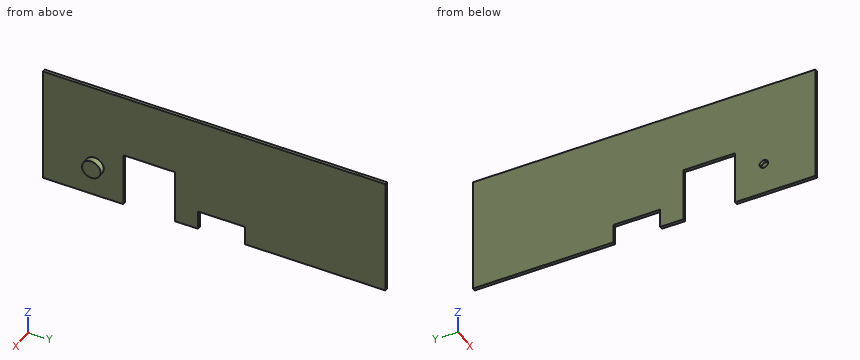
```python
from build123d import *

# Parameters (mm, degrees)
SKETCH_1_W          = 110.7
SKETCH_1_H          = 38.85
EXTRUDE_1_DEPTH     = 0.5
SKETCH_2_W          = 38.85
SKETCH_2_H          = 110.7
EXTRUDE_2_DEPTH     = 0.5
SKETCH_3_W          = 17.932827047
SKETCH_3_H          = 16.708777413
CUT_EXTRUDE_1_DEPTH = 10
SKETCH_4_W          = 6.338485403
SKETCH_4_H          = 15.09561221
CUT_EXTRUDE_2_DEPTH = 3
SKETCH_5_R          = 1.379738623
CUT_EXTRUDE_3_DEPTH = 3
SKETCH_6_R          = 3.000043017
SKETCH_6_R_2        = 2.273503066
EXTRUDE_3_DEPTH     = 1
SKETCH_7_R          = 3.000043017
EXTRUDE_4_DEPTH     = 1


with BuildPart() as part:
    # Эскиз1 → Бобышка-Вытянуть1 (new body)
    with BuildSketch(Plane(origin=(0.5, 0, 0), x_dir=(0, -1, 0), z_dir=(-1, 0, 0))):
        with Locations((-45.5, 22.825)):
            Rectangle(SKETCH_1_W, SKETCH_1_H)
    extrude(amount=-EXTRUDE_1_DEPTH)

    # Эскиз2 → Бобышка-Вытянуть2 (add)
    with BuildSketch(Plane.ZY.offset(-0.5)):
        with Locations((22.825, 45.5)):
            Rectangle(SKETCH_2_W, SKETCH_2_H)
    extrude(amount=EXTRUDE_2_DEPTH)

    # Эскиз3 → Вырез-Вытянуть1 (cut)
    with BuildSketch(Plane.ZY):
        with Locations((12.366413524, 24.461489881)):
            Rectangle(SKETCH_3_W, SKETCH_3_H)
    extrude(amount=-CUT_EXTRUDE_1_DEPTH, mode=Mode.SUBTRACT)

    # Эскиз4 → Вырез-Вытянуть2 (cut)
    with BuildSketch(Plane.ZY):
        with Locations((6.569242702, 47.853484542)):
            Rectangle(SKETCH_4_W, SKETCH_4_H)
    extrude(amount=-CUT_EXTRUDE_2_DEPTH, mode=Mode.SUBTRACT)

    # Эскиз5 → Вырез-Вытянуть3 (cut)
    with BuildSketch(Plane.ZY):
        with Locations((13.967872297, 6.805635325)):
            Circle(SKETCH_5_R)
    extrude(amount=-CUT_EXTRUDE_3_DEPTH, mode=Mode.SUBTRACT)

    # Эскиз6 → Бобышка-Вытянуть3 (add)
    with BuildSketch(Plane(origin=(1, 0, 0), x_dir=(0, 0, -1), z_dir=(1, 0, 0))):
        with Locations(Location((-13.967872297, 6.805635325, 0), (0, 0, 180))):
            Circle(SKETCH_6_R)
        with Locations((-13.967872297, 6.805635325)):
            Circle(SKETCH_6_R_2, mode=Mode.SUBTRACT)
    extrude(amount=EXTRUDE_3_DEPTH)

    # Эскиз7 → Бобышка-Вытянуть4 (add)
    with BuildSketch(Plane(origin=(2, 0, 0), x_dir=(0, 0, -1), z_dir=(1, 0, 0))):
        with Locations(Location((-13.967872297, 6.805635325, 0), (0, 0, 180))):
            Circle(SKETCH_7_R)
    extrude(amount=EXTRUDE_4_DEPTH)


solid = part.part
```
The listing builds one solid part. Answer for the finished solid, in the listing's coordinates (mm). Coordinates: 2 decimals unless noted, no trailing zeros. Write each loop counter-clockwise with the first axis right and the second up, starting at its lowest first coordinate (ties: lowest second). Pieces come first, ordered by that corner, then holes. Notation, with made-up numbers: (16, 43.25) - (28, 43.25) arc R17 ccw to (28, 59.25) - close; hole circle Ø4 at (-35, -16.75). An arc over 180 degrees is marked (long way). One line per item, written item: value.
1) Find section A-A (y = 52). Give the vertices of the cut face in (x, z).
Geometry check:
outline: (0, 9.74) - (1, 9.74) - (1, 42.25) - (0, 42.25) - close
2) Each of these flat-tipped pins is pushed along its axis until it touches: pin 1 Ø1.5 at (y, z) = (71, 38) entering from +X; pin 2 Ø0.8 at (x, y) = (0.5, 47.5) entering from -Z; pin 3 Ø2 at (y, z) = (6.81, 13.97) entering from -X. Where does it stop, or does it pass through?
Geometry check:
pin 1: stops at x = 1
pin 2: stops at z = 9.74
pin 3: stops at x = 2
3) Find section B-B (z = 22.5). Give the vertices of the cut face in (x, y).
Geometry check:
outline: (0, -9.85) - (1, -9.85) - (1, 100.85) - (0, 100.85) - close
4) Consider line 1 along X through (y, z) = (93, 22); line 2 along Z through (x, y) = (0.55, 46.5); line 3 along Y through (x, z) = (2.4, 16). Determine where each line is inside the solid, lowest interval first. Write a range as from..to.
Geometry check:
line 1: x = 0..1
line 2: z = 9.74..42.25
line 3: y = 4.6..9.01
5) Find section C-C (x = 2.5). Give the vertices of the cut face in (y, z).
Geometry check:
outline: circle Ø6 at (6.81, 13.97)
